Work out the finished part from the listing and answer in its coordinate system (mm). A direction names the side the tool comes from. Round coordinates to 2 decimals unless told otherwise and drop trailing zeros. Write each loop counter-clockwise with the first axis right and the second up, starting at its lowest first coordinate (ties: lowest second). Pieces come first, ordered by that corner, then holes. Notation, with made-up numbers: (86, 76.25) - (117, 76.25) arc R19 ccw to (117, 113.25) - close; hole circle Ø2 at (60.25, 46.25). An arc over 180 degrees is marked (long way). Write item = value, one per line. Start each with the question number.
from build123d import *

# Parameters (mm, degrees)
SKETCH1_R               = 7.5
BOSS_EXTRUDE1_DEPTH     = 10
SKETCH2_R               = 30
BOSS_EXTRUDE2_DEPTH     = 65
CUT_EXTRUDE1_DEPTH      = 65
CUT_EXTRUDE2_DEPTH      = 30
SKETCH7_R               = 6
CUT_EXTRUDE3_DEPTH      = 13.5
CUT_EXTRUDE3_DEPTH_BACK = 48.5


with BuildPart() as part:
    # Sketch1 → Boss-Extrude1 (new body)
    with BuildSketch(Plane.XY):
        with BuildLine():
            Line((75, 15), (6.126443354, 29.36778323))
            ThreePointArc((6.126443354, 29.36778323), (0, 30), (-6.126443354, 29.36778323))
            Line((-6.126443354, 29.36778323), (-75, 15))
            ThreePointArc((-75, 15), (-90, 0), (-75, -15))
            Line((-75, -15), (-6.126443354, -29.36778323))
            ThreePointArc((-6.126443354, -29.36778323), (0, -30), (6.126443354, -29.36778323))
            Line((6.126443354, -29.36778323), (75, -15))
            ThreePointArc((75, -15), (90, 0), (75, 15))
        make_face()
        with Locations((75, 0)):
            Circle(SKETCH1_R, mode=Mode.SUBTRACT)
        with Locations((-75, 0)):
            Circle(SKETCH1_R, mode=Mode.SUBTRACT)
    extrude(amount=BOSS_EXTRUDE1_DEPTH)

    # Sketch2 → Boss-Extrude2 (add)
    with BuildSketch(Plane.XY.offset(10)):
        Circle(SKETCH2_R)
    extrude(amount=BOSS_EXTRUDE2_DEPTH)

    # Sketch3 → Cut-Extrude1 (cut)
    with BuildSketch(Plane.XY.offset(75)):
        with BuildLine():
            Line((-29.047375097, -7.5), (29.047375097, -7.5))
            ThreePointArc((29.047375097, -7.5), (30, 0), (29.047375097, 7.5))
            Line((29.047375097, 7.5), (-29.047375097, 7.5))
            ThreePointArc((-29.047375097, 7.5), (-30, 0), (-29.047375097, -7.5))
        make_face()
    extrude(amount=-CUT_EXTRUDE1_DEPTH, mode=Mode.SUBTRACT)

    # Sketch4 → Cut-Extrude2 (cut)
    with BuildSketch(Plane.XY.offset(75)):
        with BuildLine():
            Line((-24.366985862, -17.5), (24.366985862, -17.5))
            ThreePointArc((24.366985862, -17.5), (0, -30), (-24.366985862, -17.5))
        make_face()
        with BuildLine():
            Line((-24.366985862, 17.5), (24.366985862, 17.5))
            ThreePointArc((24.366985862, 17.5), (0, 30), (-24.366985862, 17.5))
        make_face()
    extrude(amount=-CUT_EXTRUDE2_DEPTH, mode=Mode.SUBTRACT)

    # Sketch7 → Cut-Extrude3 (cut, two sides)
    with BuildSketch(Plane.XZ.offset(17.5)) as cut_extrude3_sk:
        with Locations((0, 60)):
            Circle(SKETCH7_R)
    extrude(amount=CUT_EXTRUDE3_DEPTH, mode=Mode.SUBTRACT)
    extrude(cut_extrude3_sk.sketch, amount=-CUT_EXTRUDE3_DEPTH_BACK, mode=Mode.SUBTRACT)


solid = part.part
1. Which of the six approach directions +Z, -Z, +X, -X, +Y, -Y give full straight-line access (tool end or side, diameter ignored) to faces 5 (the face through (0, 7.5, 43)), 6 (the face through (-6, 17.5, 64)), 7 (the face through (-6, -17.5, 64)), 8 (the face through (-1, 0, 10))?
2. Find section D-D on z = 60. Give the vertices of the cut face in (x, y), plus the area to 3 significant figures.
3. Each of these flat-tipped pins is pushed along its axis until it touches: pin 1 (4 mm diameter, centred on x = 6, y = 22, fed in from +Z); pin 2 (1 mm diameter, centred on x = -23, z = 21, fed in from +Y); pin 3 (5 mm diameter, centred on x = -63.5, y = -7.5, fed in from +Z). Where does it stop, or does it pass through?
4. Consider line 1 (Y direction, x = 75, z = 3.75); line 2 (Z direction, x = 0, y = 15); line 3 (Z direction, x = -19, y = -18). Determine where each line is inside the solid, lowest interval first.
5. For a pull along Z with two mould halves and no side action, classify faces 1 (the face through (-4.42, 12.43, 64.06)), 2 (the face through (0, -12, 75)), 3 (the face through (0, -7.5, 43)), 4 (the face through (-4.42, -12.57, 64.06)) as released by +Z, released by -Z, zero draft, split by the parting line, or undercut.
6. Find section C-C on x = 0. Give the vertices of the cut face in (y, z).
7. Find section A-A on y = 0. Give the vertices of the cut face in (x, z).
8. Find section B-B on z = 68.5. Give the vertices of the cut face in (x, y), plus the area to 3 significant figures.
Answer key:
q1.face_5 = +Z, +X, -X
q1.face_6 = +Z, +X, -X, +Y
q1.face_7 = +Z, +X, -X, -Y
q1.face_8 = +Z
q2.outline = (-29.05, -7.5) arc R30 ccw to (-24.37, -17.5) - (-6, -17.5) - (-6, -7.5) - close; (-29.05, 7.5) - (-6, 7.5) - (-6, 17.5) - (-24.37, 17.5) arc R30 ccw to start; (6, -17.5) - (24.37, -17.5) arc R30 ccw to (29.05, -7.5) - (6, -7.5) - close; (6, 7.5) - (29.05, 7.5) arc R30 ccw to (24.37, 17.5) - (6, 17.5) - close
q2.area = 843 mm²
q3.pin_1 = 45
q3.pin_2 = 19.84
q3.pin_3 = 10
q4.line_1 = -15 to -7.5, 7.5 to 15
q4.line_2 = 0 to 54, 66 to 75
q4.line_3 = 0 to 45
q5.face_1 = undercut
q5.face_2 = released by +Z
q5.face_3 = zero draft
q5.face_4 = undercut
q6.outline = (-30, 0) - (30, 0) - (30, 45) - (17.5, 45) - (17.5, 54) - (7.5, 54) - (7.5, 10) - (-7.5, 10) - (-7.5, 54) - (-17.5, 54) - (-17.5, 45) - (-30, 45) - close; (-17.5, 66) - (-7.5, 66) - (-7.5, 75) - (-17.5, 75) - close; (7.5, 66) - (17.5, 66) - (17.5, 75) - (7.5, 75) - close
q7.outline = (-90, 0) - (-82.5, 0) - (-82.5, 10) - (-90, 10) - close; (-67.5, 0) - (67.5, 0) - (67.5, 10) - (-67.5, 10) - close; (82.5, 0) - (90, 0) - (90, 10) - (82.5, 10) - close
q8.outline = (-29.05, -7.5) arc R30 ccw to (-24.37, -17.5) - (24.37, -17.5) arc R30 ccw to (29.05, -7.5) - close; (-29.05, 7.5) - (29.05, 7.5) arc R30 ccw to (24.37, 17.5) - (-24.37, 17.5) arc R30 ccw to start
q8.area = 1,080 mm²
